from build123d import *

# Parameters (mm, degrees)
EXTRU_MINCE1_DEPTH = 0.2
EXTRUSION1_DEPTH   = 0.2


with BuildPart() as part:
    # Esquisse2 → Extru.-Mince1 (new body)
    with BuildSketch(Plane.XY):
        with BuildLine():
            Line((-68.020160179, 174.136090676), (-68.020160179, 125.41885319))
            ThreePointArc((-68.020160179, 125.41885319), (-65.568146462, 116.906975155), (-58.963651719, 111.004002333))
            Line((-58.963651719, 111.004002333), (-11.723955687, 88.249106497))
            ThreePointArc((-11.723955686, 88.249106497), (-10.072832001, 86.773363292), (-9.459828571, 84.645393783))
            Line((-9.459828571, 84.645393783), (-9.459828571, -84.851832415))
            ThreePointArc((-9.459828571, -84.851832415), (-7.007814854, -93.36371045), (-0.403320111, -99.266683272))
            Line((-0.403320111, -99.266683272), (168.46168003, -180.607288974))
            ThreePointArc((168.46168003, -180.607288974), (170.112803715, -182.083032179), (170.725807145, -184.211001688))
            Line((170.725807145, -184.211001688), (170.725807145, -207.928239175))
            Line((170.725807145, -207.928239175), (182.725807145, -207.928239175))
            Line((182.725807145, -207.928239175), (182.725807145, -184.211001688))
            ThreePointArc((182.725807145, -184.211001688), (180.273793427, -175.699123653), (173.669298684, -169.796150831))
            Line((173.669298684, -169.796150831), (4.804298544, -88.455545129))
            ThreePointArc((4.804298544, -88.455545129), (3.153174858, -86.979801923), (2.540171429, -84.851832415))
            Line((2.540171429, -84.851832415), (2.540171429, 84.645393783))
            ThreePointArc((2.540171429, 84.645393783), (0.088157711, 93.157271818), (-6.516337032, 99.06024464))
            Line((-6.516337032, 99.06024464), (-53.756033064, 121.815140475))
            ThreePointArc((-53.756033064, 121.815140475), (-55.40715675, 123.290883681), (-56.020160179, 125.41885319))
            Line((-56.020160179, 125.41885319), (-56.020160179, 174.136090676))
            Line((-56.020160179, 174.136090676), (-68.020160179, 174.136090676))
        make_face()
    extrude(amount=EXTRU_MINCE1_DEPTH)

    # Esquisse3 → Extrusion1 (add)
    with BuildSketch(Plane(origin=(0, 0, 0), x_dir=(-1, 0, 0), z_dir=(0, 0, -1))):
        Polygon((-182.725807145, -207.928239175), (-194.225807145, -197.928239175), (-176.725807145, -237.928239175), (-159.225807145, -197.928239175), (-170.725807145, -207.928239175), align=None)
    extrude(amount=-EXTRUSION1_DEPTH)


solid = part.part
Input: part model. Units: mm. Frame: model coordinates. Round coordinates to 2 decimals unless told otherwise and drop trailing zeros. Loops run counter-clockwise (first coordinate to the right, second up) from the corner with the lowest first, then second, coordinate; pieces in that order, holes last. Notation, with made-up numbers: (37.5, 70.25) -> (94.5, 70.25) arc R26 cw to (94.5, 107.25) -> close; hole circle Ø3 at (70, 87). An arc over 180 degrees is marked (long way). Answer as a JSON object with one key per item and string values. Group by question number.
1) Section query A-A on z = 0.15. Output: boundary loops of the cut face in (x, y), plus the area to 3 significant figures.
2) Section query B-B on y = -64.5. Output: boundary loops of the cut face in (x, z).
3) Ray query, L1, parallel to X at y = -6.5, z = 0.15; L2, parallel to X at y = -168.5, z = 0.1; L3, parallel to Y at x = 173, z = 0.1. Return the intervals inside material, ascending.
4) Section query C-C on x = 116.5. Output: boundary loops of the cut face in (y, z), plus the area to 3 significant figures.
Reply:
{
 "1": {"outline": "(-68.02, 125.42) arc R16 ccw to (-58.96, 111) -> (-11.72, 88.25) arc R4 cw to (-9.46, 84.65) -> (-9.46, -84.85) arc R16 ccw to (-0.4, -99.27) -> (168.46, -180.61) arc R4 cw to (170.73, -184.21) -> (170.73, -207.93) -> (159.23, -197.93) -> (176.73, -237.93) -> (194.23, -197.93) -> (182.73, -207.93) -> (182.73, -184.21) arc R16 ccw to (173.67, -169.8) -> (4.8, -88.46) arc R4 cw to (2.54, -84.85) -> (2.54, 84.65) arc R16 ccw to (-6.52, 99.06) -> (-53.76, 121.82) arc R4 cw to (-56.02, 125.42) -> (-56.02, 174.14) -> (-68.02, 174.14) -> close", "area": "6,790 mm2"},
 "2": {"outline": "(-9.46, 0) -> (2.54, 0) -> (2.54, 0.2) -> (-9.46, 0.2) -> close"},
 "3": {"L1": "x = -9.46 to 2.54", "L2": "x = 143.33 to 170.98", "L3": "y = -229.41 to -169.47"},
 "4": {"outline": "(-155.58, 0) -> (-142.26, 0) -> (-142.26, 0.2) -> (-155.58, 0.2) -> close", "area": "2.66 mm2"}
}
